```python
from build123d import *

# Parameters (mm, degrees)
EXTRUDE_1_DEPTH          = 20
CUT_EXTRUDE_START        = 30
SKETCH_2_W               = 17.5
SKETCH_2_H               = 16.6
CUT_EXTRUDE_1_DEPTH      = 27.5
CUT_EXTRUDE_START_2      = 17.5
SKETCH_3_R               = 2
CUT_EXTRUDE_2_DEPTH      = 2.5
EXTRUDE_3_REACH          = 42.434
CUT_EXTRUDE_4_DEPTH      = 42.231056256
CUT_EXTRUDE_4_DEPTH_BACK = 2
SKETCH_3_2_R             = 2
CUT_EXTRUDE_6_DEPTH      = 42.231056256
CUT_EXTRUDE_6_DEPTH_BACK = 9
SKETCH_4_R               = 1.7
SKETCH_7_W               = 15.3
SKETCH_7_H               = 16.6
SKETCH_7_R               = 1.7
EXTRUDE_4_DEPTH          = 2
EXTRUDE_5_DEPTH          = 2
EXTRUDE_START            = -20
EXTRUDE_6_DEPTH          = 2


with BuildPart() as part:
    # 草图1 → 凸台-拉伸1 (new body)
    with BuildSketch(Plane.XY):
        Polygon((0, 0), (20, 0), (20, 30), (17.5, 30), (0, 2.5), align=None)
    extrude(amount=-EXTRUDE_1_DEPTH)

    # 草图2 → 切除-拉伸1 (cut)
    with BuildSketch(Plane(origin=(0, 0, 0), x_dir=(1, 0, 0), z_dir=(0, 1, 0)).offset(CUT_EXTRUDE_START)):
        with Locations((8.75, 10)):
            Rectangle(SKETCH_2_W, SKETCH_2_H)
    extrude(amount=-CUT_EXTRUDE_1_DEPTH, mode=Mode.SUBTRACT)

    # 草图3 → 切除-拉伸2 (cut)
    with BuildSketch(Plane(origin=(0, 0, 0), x_dir=(0, 0, -1), z_dir=(1, 0, 0)).offset(CUT_EXTRUDE_START_2)):
        with Locations(Location((10, 22, 0), (0, 0, 180))):
            Circle(SKETCH_3_R)
        with Locations(Location((10, 10, 0), (0, 0, 180))):
            Circle(SKETCH_3_R)
    extrude(amount=CUT_EXTRUDE_2_DEPTH, mode=Mode.SUBTRACT)

    # 草图6 → 凸台-拉伸3 (add, up to next)
    with BuildSketch(Plane(origin=(0, 0, -1.7), x_dir=(-1, 0, 0), z_dir=(0, 0, -1)), mode=Mode.PRIVATE) as extrude_3_sk1:
        Polygon((-15.3, 26.542857143), (-15.3, 2.5), (-17.5, 2.5), (-17.5, 30), align=None)
    extrude_3_tool1 = extrude(extrude_3_sk1.sketch, amount=EXTRUDE_3_REACH, mode=Mode.PRIVATE) - part.part
    add(extrude_3_tool1.solids().sort_by_distance((16.424593, 15.405038, -1.7))[0])

    # 草图3<2> → 切除-拉伸4 (cut, two sides: drawn at the far end of the back side and taken through both)
    with BuildSketch(Plane(origin=(0, 0, 0), x_dir=(0, 0, -1), z_dir=(1, 0, 0)).offset(-CUT_EXTRUDE_4_DEPTH_BACK)):
        with Locations((10, 22)):
            Circle(SKETCH_3_2_R)
        with Locations((10, 10)):
            Circle(SKETCH_3_2_R)
    extrude(amount=CUT_EXTRUDE_4_DEPTH + CUT_EXTRUDE_4_DEPTH_BACK, mode=Mode.SUBTRACT)

    # 草图4 → 切除-拉伸6 (cut, two sides: drawn at the far end of the back side and taken through both)
    with BuildSketch(Plane(origin=(0, 0, 0), x_dir=(1, 0, 0), z_dir=(0, 1, 0)).offset(-CUT_EXTRUDE_6_DEPTH_BACK)):
        with Locations(Location((9, 10, 0), (0, 0, 90))):
            Circle(SKETCH_4_R)
    extrude(amount=CUT_EXTRUDE_6_DEPTH + CUT_EXTRUDE_6_DEPTH_BACK, mode=Mode.SUBTRACT)

    # 草图7 → 凸台-拉伸4 (add)
    with BuildSketch(Plane(origin=(0, 2.5, 0), x_dir=(1, 0, 0), z_dir=(0, 1, 0))):
        with Locations((7.65, 10)):
            Rectangle(SKETCH_7_W, SKETCH_7_H)
        with Locations(Location((9, 10, 0), (0, 0, 90))):
            Circle(SKETCH_7_R, mode=Mode.SUBTRACT)
    extrude(amount=EXTRUDE_4_DEPTH)

    # 草图8 → 凸台-拉伸5 (add)
    with BuildSketch(Plane(origin=(0, 0, -20), x_dir=(-1, 0, 0), z_dir=(0, 0, -1))):
        Polygon((0, 0), (0, 2.5), (-17.5, 30), (-20, 30), (-20, 0), align=None)
    extrude(amount=EXTRUDE_5_DEPTH)

    # 草图8<2> → 凸台-拉伸6 (add)
    with BuildSketch(Plane(origin=(0, 0, -20), x_dir=(-1, 0, 0), z_dir=(0, 0, -1)).offset(EXTRUDE_START)):
        Polygon((0, 0), (0, 2.5), (-17.5, 30), (-20, 30), (-20, 0), align=None)
    extrude(amount=-EXTRUDE_6_DEPTH)


solid = part.part
```
Model file for the job. Use its own axes, mm. A direction names the side the tool comes from. Coordinates: 2 decimals unless noted, no trailing zeros. Loops run counter-clockwise (first coordinate to the right, second up) from the corner with the lowest first, then second, coordinate; pieces in that order, holes last. Notation, with made-up numbers: (38, -40) - (48, -40) arc R29 ccw to (48, -3) - close; hole circle Ø11 at (-6, 45.5). An arc over 180 degrees is marked (long way). Write item = value, one per line. Start each with the question number.
Item 1: Pull direction Y, two halves, no side cores. Call faces 1 (the face through (12, 0, -10)), 2 (the face through (17, 24, -10)), 3 (the face through (6, 4.5, -10)): +Y half, -Y half, draft (parallel to the pull), parting line (faces both ways), or undercut.
Item 2: Saw through at B-B, the plane y = 24.5. List the corners of the cut face in (x, z), then the cut area to 3 significant figures.
Item 3: Saw through at D-D, the plane y = 21.5. List the corners of the cut face in (x, z).
Item 4: Wall check: probe 1 along Z at (x, y) = (18.45, 10); probe 2 along X at (y, z) = (1.05, -10); probe 3 along Z at (x, y) = (9, 2.8). Give the ranges that are in metal, low to high. Write a range as [from, to].
Item 5: 3-axis set-ups, long thin cutter, end or side, ignore diameter. For faces 4 (the face through (0.3, 3.9, -18.3)), 5 (the face through (0, 2, -10)), 6 (the face through (11, 11, -1.7)), 7 (the face through (10.66, 2.22, -9.63)), 8 (the face through (0.3, 3.9, -1.7)): which of +Z, -Z, +X, -X, +Y, -Y reach the whole face in a straight line?
Item 6: Saw through at A-A, the plane z = -10. List the corners of the cut face in (x, y), then the cut area to 3 significant figures.
Item 7: Saw through at C-C, the plane x = 14. List the corners of the cut face in (y, z), then the cut area to 3 significant figures.
Item 8: Drop flat-ended pins along their axis: pin 1 Ø3 at (y, z) = (9.5, -18) entering from -X; pin 2 Ø10 at (y, z) = (23, -3) entering from -X; pin 3 Ø8.5 at (y, z) = (10.5, -7) entering from -X; pin 4 Ø2.5 at (x, z) = (9, -10) entering from +Y. Give the stop position or say it passes through.
Answers:
q1.face_1 = -Y half
q1.face_2 = undercut
q1.face_3 = +Y half
q2.outline = (14, -22) - (20, -22) - (20, 2) - (14, 2) - (14, -1.7) - (15.3, -1.7) - (15.3, -18.3) - (14, -18.3) - close
q2.area = 122 mm2
q3.outline = (12.09, -22) - (20, -22) - (20, -11.94) - (15.3, -11.94) - (15.3, -18.3) - (12.09, -18.3) - close; (12.09, -1.7) - (15.3, -1.7) - (15.3, -8.06) - (20, -8.06) - (20, 2) - (12.09, 2) - close
q4.probe_1 = [-22, -12], [-8, 2]
q4.probe_2 = [0, 7.3], [10.7, 20]
q4.probe_3 = [-22, -11.7], [-8.3, 2]
q5.face_4 = -Z, -X, +Y
q5.face_5 = +Z, -Z, -X, +Y, -Y
q5.face_6 = -X, +Y
q5.face_7 = +Y, -Y
q5.face_8 = +Z, -X, +Y
q6.outline = (0, 0) - (7.3, 0) - (7.3, 4.5) - (0, 4.5) - close; (10.7, 0) - (20, 0) - (20, 8) - (15.3, 8) - (15.3, 4.5) - (10.7, 4.5) - close; (15.3, 12) - (20, 12) - (20, 20) - (15.3, 20) - close; (15.3, 24) - (20, 24) - (20, 30) - (17.5, 30) - (15.3, 26.54) - close
q6.area = 153 mm2
q7.outline = (0, -22) - (24.5, -22) - (24.5, -18.3) - (4.5, -18.3) - (4.5, -1.7) - (24.5, -1.7) - (24.5, 2) - (0, 2) - close
q7.area = 256 mm2
q8.pin_1 = 3.52
q8.pin_2 = 9.97
q8.pin_3 = 15.3
q8.pin_4 = through
